from build123d import *

# Parameters (mm, degrees)
F1_DEPTH = 25
F3_R     = 2.5
F4_DEPTH = 25
F2_R     = 2.5
F5_DEPTH = 25


# Not quite as in the source:
# - ends of sketch curves that miss each other by under 0.0002 mm in the source are joined


with BuildPart() as f1:
    # F0 (on Front) → F1 (new body)
    with BuildSketch(Plane.XZ):
        with BuildLine():
            Line((-47.4549531937, 57.8603595495), (47.4549531937, 57.8603595495))
            Line((47.4549531937, 57.8603595495), (47.4549531937, 65.1126131415))
            Line((47.4549531937, 65.1126131415), (-47.4549531937, 65.1126131415))
            ThreePointArc((-47.4549531937, 65.1126131415), (-52.5830735216, 62.9884798775), (-54.707210511, 57.8603595495))
            Line((-54.707210511, 57.8603595495), (-54.7072067857, -57.8603595495))
            ThreePointArc((-54.7072067857, -57.8603595495), (-52.5830708875, -62.9884772433), (-47.4549531937, -65.1126131415))
            Line((-47.4549531937, -65.1126131415), (-47.4549531937, -57.8603595495))
            Line((-47.4549531937, -57.8603595495), (-47.4549531937, 57.8603595495))
        make_face()
        with BuildLine():
            Line((47.4549531937, 65.1126131415), (47.4549531937, 57.8603595495))
            Line((47.4549531937, 57.8603595495), (47.4549531937, -57.8603595495))
            Line((47.4549531937, -57.8603595495), (-47.4549531937, -57.8603595495))
            Line((-47.4549531937, -57.8603595495), (-47.4549531937, -65.1126131415))
            Line((-47.4549531937, -65.1126131415), (47.4549531937, -65.1126131415))
            ThreePointArc((47.4549531937, -65.1126131415), (52.5830735216, -62.9884798775), (54.707210511, -57.8603595495))
            Line((54.707210511, -57.8603595495), (54.7072067857, 57.8603595495))
            ThreePointArc((54.7072067857, 57.8603595495), (52.5830708875, 62.9884772433), (47.4549531937, 65.1126131415))
        make_face()
    extrude(amount=F1_DEPTH)

    # F3 (on face) → F4 (cut)
    with BuildSketch(Plane(origin=(0, 0, -65.1126131415), x_dir=(1, 0, 0), z_dir=(0, 0, -1))):
        with Locations((0, 12.5)):
            Circle(F3_R)
    extrude(amount=-F4_DEPTH, mode=Mode.SUBTRACT)

    # F2 (on face) → F5 (cut)
    with BuildSketch(Plane.XY.offset(65.1126131415)):
        with Locations((0, -12.5)):
            Circle(F2_R)
    extrude(amount=-F5_DEPTH, mode=Mode.SUBTRACT)


solid = f1.part
Model file for the job. Use its own axes, mm. A direction names the side the tool comes from. Coordinates: 2 decimals unless noted, no trailing zeros. Write each loop counter-clockwise with the first axis right and the second up, starting at its lowest first coordinate (ties: lowest second). Pieces come first, ordered by that corner, then holes. Notation, with made-up numbers: (70.25, -33) -> (74.25, -33) arc R11 ccw to (74.25, -29) -> close; hole circle Ø2 at (53, 83.25). An arc over 180 degrees is marked (long way). One line per item, written item: value. Start each with the question number.
1) Slice it at C-C on y = -12.5. Write the cut outline in (x, z), then the cut area to 3 significant figures.
2) Pull direction X, two halves, no side cores. Call faces 1 (the face through (-54.707, -12, 1)), 2 (the face through (1, -10, 65.113)), 3 (the face through (1, -10, -57.86)): +X half, -X half, draft (parallel to the pull), parting line (faces both ways), or undercut.
3) Slice it at D-D on x = -46. Write the cut outline in (y, z), then the cut area to 3 significant figures.
4) Probe probe 1 along Z at (x, y) = (4, -3.5); probe 2 along Y at (x, z) = (0, 59.5); probe 3 along X at (y, z) = (-20.75, -22.5). List the from-to ranges inside material, lowest first.
5) Slice it at A-A on x = 0. Write the cut outline in (y, z), then the cut area to 3 significant figures.
6) Which spindle directions (+Z, -Z, +X, -X, +Y, -Y) get a long thin tool onto all of the face, cutting with end or side? Do faces 4 (the face through (-1, -10, 57.86)), 5 (the face through (-1, -10, -65.113)). Say none if no direction does.
7) Slice it at B-B on z = -42. Write the cut outline in (x, y), then the cut area to 3 significant figures.
Answers follow:
1. outline: (-54.71, -57.86) arc R7.25 ccw to (-47.45, -65.11) -> (-2.5, -65.11) -> (-2.5, -57.86) -> (-47.45, -57.86) -> (-47.45, 57.86) -> (-2.5, 57.86) -> (-2.5, 65.11) -> (-47.45, 65.11) arc R7.25 ccw to (-54.71, 57.86) -> close; (2.5, -65.11) -> (47.45, -65.11) arc R7.25 ccw to (54.71, -57.86) -> (54.71, 57.86) arc R7.25 ccw to (47.45, 65.11) -> (2.5, 65.11) -> (2.5, 57.86) -> (47.45, 57.86) -> (47.45, -57.86) -> (2.5, -57.86) -> close
1. area: 3,150 mm2
2. face 1: -X half
2. face 2: draft
2. face 3: undercut
3. outline: (-25, -65.11) -> (0, -65.11) -> (0, -57.86) -> (-25, -57.86) -> close; (-25, 57.86) -> (0, 57.86) -> (0, 65.11) -> (-25, 65.11) -> close
3. area: 363 mm2
4. probe 1: -65.11 to -57.86, 57.86 to 65.11
4. probe 2: -25 to -15, -10 to 0
4. probe 3: -54.71 to -47.45, 47.45 to 54.71
5. outline: (-25, -65.11) -> (-15, -65.11) -> (-15, -57.86) -> (-25, -57.86) -> close; (-25, 57.86) -> (-15, 57.86) -> (-15, 65.11) -> (-25, 65.11) -> close; (-10, -65.11) -> (0, -65.11) -> (0, -57.86) -> (-10, -57.86) -> close; (-10, 57.86) -> (0, 57.86) -> (0, 65.11) -> (-10, 65.11) -> close
5. area: 290 mm2
6. face 4: +Y, -Y
6. face 5: -Z, +X, -X, +Y, -Y
7. outline: (-54.71, -25) -> (-47.45, -25) -> (-47.45, 0) -> (-54.71, 0) -> close; (47.45, -25) -> (54.71, -25) -> (54.71, 0) -> (47.45, 0) -> close
7. area: 363 mm2
